```python
from build123d import *

# Parameters (mm, degrees)
SKETCH_1_W      = 25
SKETCH_1_H      = 3
SKETCH_1_R      = 1.55
EXTRUDE_1_DEPTH = 3
FILLET_2_R      = 3
FILLET_4_R      = 2
FILLET_5_R      = 1.5
FILLET_6_R      = 3
FILLET_1_R      = 2


with BuildPart() as part:
    # 草图1 → 凸台-拉伸1 (new body)
    with BuildSketch(Plane.XY):
        with BuildLine():
            Line((-34.5, 31), (-45.5, 31))
            Line((-45.5, 31), (-45.5, 21))
            Line((-45.5, 21), (-30, 21))
            Line((-30, 21), (-30, 6))
            Line((-30, 6), (-45.5, 6))
            Line((-45.5, 6), (-45.5, -3))
            Line((-45.5, -3), (-30, -3))
            Line((-30, -3), (-30, -6.9))
            ThreePointArc((-30, -6.9), (-28.95, -7.95), (-30, -9))
            Line((-30, -9), (-33, -9))
            Line((-33, -9), (-33, -19))
            Line((-33, -19), (-30, -19))
            ThreePointArc((-30, -19), (-28.95, -20.05), (-30, -21.1))
            Line((-30, -21.1), (-30, -28))
            Line((-30, -28), (-20.5, -28))
            Line((-20.5, -28), (-17.5, -31))
            Line((-17.5, -31), (-17.5, -35))
            Line((-17.5, -35), (17.5, -35))
            Line((17.5, -35), (17.5, -31))
            Line((17.5, -31), (20.5, -28))
            Line((20.5, -28), (30, -28))
            Line((30, -28), (30, -15.5))
            Line((30, -15.5), (33, -12.5))
            Line((33, -12.5), (33, 12.5))
            Line((33, 12.5), (30, 15.5))
            Line((30, 15.5), (30, 28))
            Line((30, 28), (17.5, 28))
            Line((17.5, 28), (17.5, 32))
            Line((17.5, 32), (-17.5, 32))
            Line((-17.5, 32), (-17.5, 28))
            Line((-17.5, 28), (-21.5, 28))
            Line((-21.5, 28), (-34.5, 31))
        make_face()
        with Locations((0, -31.5)):
            Rectangle(SKETCH_1_W, SKETCH_1_H, mode=Mode.SUBTRACT)
        with BuildLine():
            Line((25, -10.3), (25, -23))
            Line((25, -23), (11.3, -23))
            Line((11.3, -23), (11.3, -26))
            ThreePointArc((11.3, -26), (10.25, -27.05), (9.2, -26))
            Line((9.2, -26), (7.1, -26))
            ThreePointArc((7.1, -26), (6.05, -27.05), (5, -26))
            Line((5, -26), (5, -23))
            Line((5, -23), (-5, -23))
            Line((-5, -23), (-5, -26))
            ThreePointArc((-5, -26), (-6.05, -27.05), (-7.1, -26))
            Line((-7.1, -26), (-9.2, -26))
            ThreePointArc((-9.2, -26), (-10.25, -27.05), (-11.3, -26))
            Line((-11.3, -26), (-11.3, -23))
            Line((-11.3, -23), (-25, -23))
            Line((-25, -23), (-25, 23))
            Line((-25, 23), (25, 23))
            Line((25, 23), (25, 10.3))
            Line((25, 10.3), (28, 10.3))
            ThreePointArc((28, 10.3), (29.05, 9.25), (28, 8.2))
            Line((28, 8.2), (28, 6.1))
            ThreePointArc((28, 6.1), (29.05, 5.05), (28, 4))
            Line((28, 4), (25, 4))
            Line((25, 4), (25, -4))
            Line((25, -4), (28, -4))
            ThreePointArc((28, -4), (29.05, -5.05), (28, -6.1))
            Line((28, -6.1), (28, -8.2))
            ThreePointArc((28, -8.2), (29.05, -9.25), (28, -10.3))
            Line((28, -10.3), (25, -10.3))
        make_face(mode=Mode.SUBTRACT)
        with Locations((-40.5, 1)):
            Circle(SKETCH_1_R, mode=Mode.SUBTRACT)
        with Locations((-40.5, 26)):
            Circle(SKETCH_1_R, mode=Mode.SUBTRACT)
        with Locations((0, 27.5)):
            Rectangle(SKETCH_1_W, SKETCH_1_H, mode=Mode.SUBTRACT)
    extrude(amount=EXTRUDE_1_DEPTH)

    # 圆角2
    fillet_2_edges = [part.edges().sort_by_distance(p)[0] for p in [
        (30, 28, 1.5),
    ]]
    fillet(fillet_2_edges, radius=FILLET_2_R)

    # 圆角4
    fillet_4_edges = [part.edges().sort_by_distance(p)[0] for p in [
        (-30, 21, 1.5),
    ]]
    fillet(fillet_4_edges, radius=FILLET_4_R)

    # 圆角5
    fillet_5_edges = [part.edges().sort_by_distance(p)[0] for p in [
        (-45.5, -3, 1.5),
        (-45.5, 31, 1.5),
        (-34.5, 31, 1.5),
        (-21.5, 28, 1.5),
    ]]
    fillet(fillet_5_edges, radius=FILLET_5_R)

    # 圆角6
    fillet_6_edges = [part.edges().sort_by_distance(p)[0] for p in [
        (-30, -3, 1.5),
        (-30, 6, 1.5),
    ]]
    fillet(fillet_6_edges, radius=FILLET_6_R)

    # 圆角1
    fillet_1_edges = [part.edges().sort_by_distance(p)[0] for p in [
        (25, 23, 1.5),
        (-25, 23, 1.5),
        (-25, -23, 1.5),
        (25, -23, 1.5),
        (-45.5, 6, 1.5),
        (-45.5, 21, 1.5),
        (-17.5, 32, 1.5),
        (17.5, 32, 1.5),
        (17.5, 28, 1.5),
        (33, 12.5, 1.5),
        (33, -12.5, 1.5),
        (30, -28, 1.5),
        (20.5, -28, 1.5),
        (17.5, -31, 1.5),
        (17.5, -35, 1.5),
        (-17.5, -35, 1.5),
        (-30, -28, 1.5),
    ]]
    fillet(fillet_1_edges, radius=FILLET_1_R - 0.0001)  # a hair under: the kernel refuses the full size


solid = part.part
```
The model under review builds one solid part; all positions refer to its coordinate system, in mm. A direction names the side the tool comes from. Round coordinates to 2 decimals unless told otherwise and drop trailing zeros. Order: outer loops, then holes, each group sorted by start corner. A loop starts at its lowest first (then second) coordinate and runs counter-clockwise, first axis right, second up. Notation, with made-up numbers: M -21.75,-5.75 L 8.25,-5.75 A21 cw 8.25,22.25 Z; hole C 48,-25.75 d2. An arc over 180 degrees is marked long. Use a Markdown table: item, result.
1) Consider section A-A (x = -6.05). Write out the cut boundary in (y, z).
Report:
| item | result |
|---|---|
| outline | M -35,0 L -33,0 L -33,3 L -35,3 Z; M -30,0 L -27.05,0 L -27.05,3 L -30,3 Z; M 23,0 L 26,0 L 26,3 L 23,3 Z; M 29,0 L 32,0 L 32,3 L 29,3 Z |
2) Consider section C-C (x = -36.5). Write out the cut boundary in (y, z).
Report:
| item | result |
|---|---|
| outline | M -3,0 L 6,0 L 6,3 L -3,3 Z; M 21,0 L 31,0 L 31,3 L 21,3 Z |
3) Wall thickness on line 1 along Y through (x, z) = (-40.5, 0.8); line 2 along X through (y, z) = (-23.5, 1); line 3 along Y through (x, z) = (0.5, 1): over which ranges is each line inside the solid? List them lowest first. Write a range as [from, to].
Report:
| item | result |
|---|---|
| line 1 | [-3, -0.55], [2.55, 6], [21, 24.45], [27.55, 31] |
| line 2 | [-30, -11.3], [-5, 5], [11.3, 30] |
| line 3 | [-35, -33], [-30, -23], [23, 26], [29, 32] |
4) Tool access review of faces 5 (the face through (12.5, 27, 1)), 6 (the face through (29.43, -27.4, 1.52)), 7 (the face through (30, 20, 1)), 8 (the face through (-30.6, 20.43, 1.52)): name each direction out of +Z, -Z, +X, -X, +Y, -Y from which nothing blocks a thin tool from reaching the whole face with its end or side.
Report:
| item | result |
|---|---|
| face 5 | +Z, -Z |
| face 6 | +Z, -Z, +X, -Y |
| face 7 | +Z, -Z, +X, +Y |
| face 8 | +Z, -Z, -X |
5) Draft analysis for pull direction Y (two halves, no side actions). For faces 1 (the face through (0, 32, 1)), 2 (the face through (-39, -3, 1)), 3 (the face through (-17.5, 29, 1)), 4 (the face through (-12.5, 27, 1)), state which applies: released by +Y, released by -Y, zero draft, split by the parting line, or undercut.
Report:
| item | result |
|---|---|
| face 1 | released by +Y |
| face 2 | released by -Y |
| face 3 | zero draft |
| face 4 | undercut |
6) Insertion check: pin 1 (1.5 mm diameter, centred on y = 15.5, z = 1.5, fed in from -X); pin 2 (0.9 mm diameter, centred on x = 26, z = 2, fed in from -Y); pin 3 (0.6 mm diameter, centred on y = -7.5, z = 2, fed in from -X). Each pin has a flat end and moves straight along its axis. Give the tip position at first contact, or say it passes through.
Report:
| item | result |
|---|---|
| pin 1 | x = -30 |
| pin 2 | y = -28 |
| pin 3 | x = -29.27 |
7) Consider section D-D (z = 2.2). Give the number of separate pieces and of enclosed holes in the cut face, then the cut area to 3 significant figures.
Report:
| item | result |
|---|---|
| separate pieces | 1 |
| enclosed holes | 5 |
| area | 1,610 mm^2 |
8) Consider section B-B (y = 18). Write out the cut boundary in (x, z).
Report:
| item | result |
|---|---|
| outline | M -30,0 L -25,0 L -25,3 L -30,3 Z; M 25,0 L 30,0 L 30,3 L 25,3 Z |
